Input: part model. Units: mm. Frame: model coordinates. A direction names the side the tool comes from. Give positions to 0.01 mm unless a question says otherwise; leave off trailing zeros. Loops run counter-clockwise (first coordinate to the right, second up) from the corner with the lowest first, then second, coordinate; pieces in that order, holes last. Notation, with made-up numbers: (50.5, 55.25) - (65.5, 55.25) arc R17 ccw to (65.5, 80.25) - close; hole circle Ø2 at (4.5, 32.25). An arc over 180 degrees is marked (long way). Answer as a JSON object with one key per item and string values. Group by question number.
(1) Section query A-A (y = -1.75). Return loops of the section in (x, z).
(2) Pin query (flat end, axial travel): P1, Ø0.9, axis at x = 0, z = 1.5, coming from the +Y side; P2, Ø4, axis at x = -3, y = -2.5, coming from the -Z side; P3, Ø1.9, axis at x = 0, y = 5.5, coming from the +Z side. Return the tip coordinate at first contact, or that it passes through.
(3) Mould query, pull axis X, two halves, no side actions, for faces 3 (the flat face through (0, -4, 1)), 4 (the flat face through (0, 5, -0.5)), 5 (the cylindrical face through (2, 0, 1)). Classes: +X half, -X half, draft (parallel to the pull), parting line (faces both ways), or undercut.
(4) Material intervals for L1, parallel to X at y = 5.5, z = 0.75; L2, parallel to Z at x = -1.25, y = 4.5; L3, parallel to Y at x = -0.25, z = 0.5, sorted ascending.
(5) Access query for faces 1 (the flat face through (1.293, 4.986, 1.76)), 2 (the flat face through (2, 4, 3)). Directions: +Z, -Z, +X, -X, +Y, -Y. A direction counts if a zero-diameter tool reaches every point of the face in a straight line with its end or side. Return the directions, or none.
```python
from build123d import *

# Parameters (mm, degrees)
SKETCH15_W           = 2
SKETCH15_H           = 8
SKETCH19_R           = 1.75
BOSS_EXTRUDE11_DEPTH = 2


with BuildPart() as part:
    # Sketch15 → Revolve3 (revolve)
    with BuildSketch(Plane(origin=(0, 0, 0), x_dir=(0, 0, -1), z_dir=(1, 0, 0))):
        Rectangle(SKETCH15_W, SKETCH15_H)
        with BuildLine():
            Line((0.75, 6), (0.75, 4))
            Line((0.75, 4), (1, 4))
            Line((1, 4), (2.75, 4))
            add(Edge.make_bspline(
                [(0.75, 6), (2.290975881, 5.319572534), (2.75, 4)],
                knots=[0, 0, 0, 0.856055689, 0.856055689, 0.856055689], degree=2))
        make_face()
    revolve(axis=Axis((0, -4, 1), (0, 1, 0)))

    # Sketch19 → Boss-Extrude11 (add)
    with BuildSketch(Plane(origin=(0, 4, 0), x_dir=(1, 0, 0), z_dir=(0, 1, 0))):
        with Locations((0, -1)):
            Circle(SKETCH19_R)
        Polygon((1.732050808, -1), (0.866025404, 0.5), (-0.866025404, 0.5), (-1.732050808, -1), (-0.866025404, -2.5), (0.866025404, -2.5), align=None, mode=Mode.SUBTRACT)
    extrude(amount=BOSS_EXTRUDE11_DEPTH)


solid = part.part
```
Recorded:
{
 "1": {"outline": "circle Ø4 at (0, 1)"},
 "2": {"P1": "stops at y = 4", "P2": "stops at z = -0.73", "P3": "stops at z = 4.5"},
 "3": {"face 3": "draft", "face 4": "undercut", "face 5": "parting line"},
 "4": {"L1": "x = -2.61 to -1.59, 1.59 to 2.61", "L2": "z = -2.3 to 0.17, 1.83 to 4.3", "L3": "y = -4 to 4"},
 "5": {"face 1": "+Y", "face 2": "-Y"}
}
